Check sheet for the modelled part. Datum: model origin and axes. Units: mm. Face numbers are marked on the shaded views. Give positions to 0.01 mm unless a question says otherwise; leave off trailing zeros. Order: outer loops, then holes, each group sorted by start corner. A loop starts at its lowest first (then second) coordinate and runs counter-clockwise, first axis right, second up. Notation, with made-up numbers: (-30, 85) -> (14, 85) arc R24 ccw to (14, 123) -> close; hole circle Ø7 at (-35, 11). An arc over 180 degrees is marked (long way). One line per question, with ' | ' between items.
```python
from build123d import *

# Parameters (mm, degrees)
F0_R     = 14
F0_R_2   = 12
F1_DEPTH = 16
F3_DEPTH = 2.5
F4_R     = 14
F5_DEPTH = 3
F6_R     = 2


with BuildPart() as f1:
    # F0 (on Top) → F1 (new body)
    with BuildSketch(Plane.XY):
        Circle(F0_R)
        Circle(F0_R_2, mode=Mode.SUBTRACT)
    extrude(amount=F1_DEPTH)

    # F2 (on Top) → F3 (join)
    with BuildSketch(Plane.XY):
        with BuildLine():
            Line((-11.2159206042, 0.875), (-11.968056442, 0.875))
            ThreePointArc((-11.968056442, 0.875), (-12, 0), (-11.968056442, -0.875))
            Line((-11.968056442, -0.875), (-11.2159206042, -0.875))
            ThreePointArc((-11.2159206042, -0.875), (-11.25, 0), (-11.2159206042, 0.875))
        make_face()
        with BuildLine():
            ThreePointArc((11.968056442, -0.875), (12, 0), (11.968056442, 0.875))
            Line((11.968056442, 0.875), (11.2159206042, 0.875))
            ThreePointArc((11.2159206042, 0.875), (11.25, 0), (11.2159206042, -0.875))
            Line((11.2159206042, -0.875), (11.968056442, -0.875))
        make_face()
    extrude(amount=F3_DEPTH)

    # F4 (on face) → F5 (join)
    with BuildSketch(Plane.XY.offset(16)):
        Circle(F4_R)
    extrude(amount=F5_DEPTH)

    # F6
    f6_edges = [f1.edges().sort_by_distance(p)[0] for p in [
        (-14, 0, 19),
    ]]
    fillet(f6_edges, radius=F6_R)


solid = f1.part
```
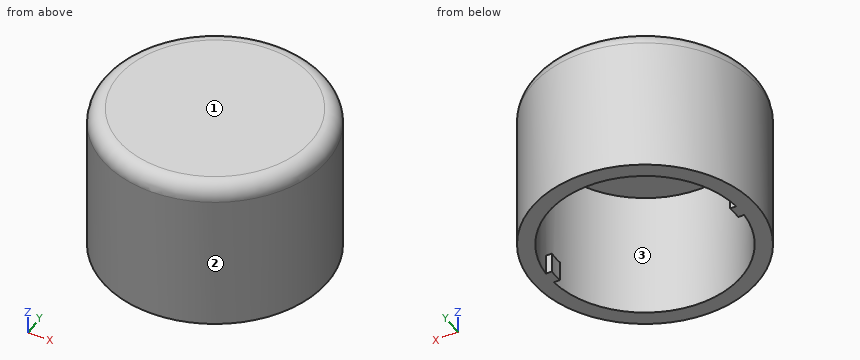
Q1. Section check C-C (z = 6.5). Enter the section's corners in (x, y).
Result sheet:
outline: circle Ø28 at (0, 0); hole circle Ø24 at (0, 0)
Q2. Thickness scan on line 1 (Y direction, x = 0, z = 7.75); line 2 (Z direction, x = -4.75, y = 5); line 3 (Y direction, x = -7.5, z = 11.75). Record the ranges inside material, lowest first.
Result sheet:
line 1: y = -14 to -12, 12 to 14 | line 2: z = 16 to 19 | line 3: y = -11.82 to -9.37, 9.37 to 11.82
Q3. Section check A-A (y = 0). Enter the section's corners in (x, z), and give its area (3 significant figures).
Result sheet:
outline: (-14, 0) -> (-11.25, 0) -> (-11.25, 2.5) -> (-12, 2.5) -> (-12, 16) -> (12, 16) -> (12, 2.5) -> (11.25, 2.5) -> (11.25, 0) -> (14, 0) -> (14, 17) arc R2 ccw to (12, 19) -> (-12, 19) arc R2 ccw to (-14, 17) -> close | area: 150 mm2
Q4. Depth check by flat-ended pin: pin 1 Ø3 at (x, z) = (-10, 17) entering from +Y; pin 2 Ø1.5 at (x, y) = (-5.5, 3) entering from -Z; pin 3 Ø0.8 at (x, z) = (-11.5, 1) entering from -Y. Enter the tip coordinate at first touch or a pass-through.
Result sheet:
pin 1: stops at y = 11.12 | pin 2: stops at z = 16 | pin 3: stops at y = -8.53
Q5. Section check B-B (z = 16.5). Enter the section's corners in (x, y).
Result sheet:
outline: circle Ø28 at (0, 0)
Q6. Mould release check, pull along X, two halves, no side actions. Record for the marked faces 1, 2 and 3: pulls with the +X half, pulls with the -X half, needs draft (parallel to the pull), parting line crosses it, or undercut.
Result sheet:
face 1: needs draft | face 2: parting line crosses it | face 3: undercut
